```python
from build123d import *

# Parameters (mm, degrees)
BOSS_EXTRUDE2_START = 10
SKETCH3_W           = 70
SKETCH3_H           = 5
BOSS_EXTRUDE2_DEPTH = 120
BOSS_EXTRUDE3_START = 18
BOSS_EXTRUDE3_DEPTH = 8
SKETCH4_R           = 2.1
CUT_EXTRUDE1_DEPTH  = 11
FILLET1_R           = 10
SKETCH5_R           = 1.6
CUT_EXTRUDE2_DEPTH  = 11
CUT_EXTRUDE5_REACH  = 139.915
SKETCH7_R           = 1.6
CUT_EXTRUDE6_REACH  = 139.915
SKETCH6_W           = 40
SKETCH6_H           = 4


with BuildPart() as part:
    # Sketch3 → Boss-Extrude2 (new body)
    with BuildSketch(Plane.XY.offset(BOSS_EXTRUDE2_START)):
        with Locations((0, 11)):
            Rectangle(SKETCH3_W, SKETCH3_H)
    extrude(amount=BOSS_EXTRUDE2_DEPTH)

    # Sketch1 → Boss-Extrude3 (add, symmetric)
    with BuildSketch(Plane.XY.offset(BOSS_EXTRUDE3_START)):
        with BuildLine():
            Line((-14.625621312, 8.5), (14.625621312, 8.5))
            add(Edge.make_bspline(
                [(14.625621312, 8.5), (12.253002272, 8.152861079), (11.086674652, 1.382068579), (9.719671925, -2.351165174)],
                knots=[0, 0, 0, 0, 1, 1, 1, 1], degree=3))
            ThreePointArc((9.719671925, -2.351165174), (9.204012528, -3.909751064), (8.440296287, -5.362965465))
            ThreePointArc((8.440296287, -5.362965465), (7.859364307, -6.648156809), (7.660444431, -8.044448198))
            Line((7.660444431, -8.044448198), (7.660444431, -16.427876097))
            Line((7.660444431, -16.427876097), (6.160444431, -16.427876097))
            Line((6.160444431, -16.427876097), (5.160444431, -16.427876097))
            Line((5.160444431, -16.427876097), (5.160444431, -6.557170147))
            ThreePointArc((5.160444431, -6.557170147), (5.34546922, -4.208445066), (5.895979032, -1.917662968))
            ThreePointArc((5.895979032, -1.917662968), (0, 6.2), (-5.895979032, -1.917662968))
            ThreePointArc((-5.895979032, -1.917662968), (-5.34546922, -4.208445066), (-5.160444431, -6.557170147))
            Line((-5.160444431, -6.557170147), (-5.160444431, -16.427876097))
            Line((-5.160444431, -16.427876097), (-6.160444431, -16.427876097))
            Line((-6.160444431, -16.427876097), (-7.660444431, -16.427876097))
            Line((-7.660444431, -16.427876097), (-7.660444431, -8.044448198))
            ThreePointArc((-7.660444431, -8.044448198), (-7.859364307, -6.648156809), (-8.440296287, -5.362965465))
            ThreePointArc((-8.440296287, -5.362965465), (-9.204012528, -3.909751064), (-9.719671925, -2.351165174))
            add(Edge.make_bspline(
                [(-14.625621312, 8.5), (-12.253002272, 8.152861079), (-11.086674652, 1.382068579), (-9.719671925, -2.351165174)],
                knots=[0, 0, 0, 0, 1, 1, 1, 1], degree=3))
        make_face()
    boss_extrude3 = extrude(amount=BOSS_EXTRUDE3_DEPTH, both=True)

    # Sketch4 → Cut-Extrude1 (cut)
    with BuildSketch(Plane.ZY.offset(7.660444431)):
        with Locations(Location((18, -12.521824291, 0), (0, 0, 270))):
            Circle(SKETCH4_R)
    cut_extrude1 = extrude(amount=-CUT_EXTRUDE1_DEPTH, mode=Mode.SUBTRACT)

    # Mirror2: Boss-Extrude3, Cut-Extrude1 across plane
    add(boss_extrude3.mirror(Plane.XY.offset(70)))
    add(cut_extrude1.mirror(Plane.XY.offset(70)), mode=Mode.SUBTRACT)

    # Fillet1
    fillet1_edges = [part.edges().sort_by_distance(p)[0] for p in [
        (-35, 11, 130),
        (35, 11, 130),
        (-35, 11, 10),
        (35, 11, 10),
    ]]
    fillet(fillet1_edges, radius=FILLET1_R)

    # Sketch5 → Cut-Extrude2 (cut)
    with BuildSketch(Plane(origin=(0, 13.5, 0), x_dir=(1, 0, 0), z_dir=(0, 1, 0))):
        with Locations(Location((29, -25, 0), (0, 0, 270))):
            Circle(SKETCH5_R)
        with Locations(Location((29, -74, 0), (0, 0, 270))):
            Circle(SKETCH5_R)
        with Locations(Location((-29, -74, 0), (0, 0, 270))):
            Circle(SKETCH5_R)
        with Locations(Location((-29, -25, 0), (0, 0, 270))):
            Circle(SKETCH5_R)
    extrude(amount=-CUT_EXTRUDE2_DEPTH, mode=Mode.SUBTRACT)

    # Sketch7 → Cut-Extrude5 (cut, up to next)
    with BuildSketch(Plane(origin=(0, 13.5, 0), x_dir=(1, 0, 0), z_dir=(0, 1, 0)), mode=Mode.PRIVATE) as cut_extrude5_sk1:
        with Locations(Location((12.5, -37, 0), (0, 0, 270))):
            Circle(SKETCH7_R)
    cut_extrude5_tool1 = extrude(cut_extrude5_sk1.sketch, amount=-CUT_EXTRUDE5_REACH, mode=Mode.PRIVATE) & part.part
    # Sketch7 → Cut-Extrude5 (cut, up to next)
    with BuildSketch(Plane(origin=(0, 13.5, 0), x_dir=(1, 0, 0), z_dir=(0, 1, 0)), mode=Mode.PRIVATE) as cut_extrude5_sk2:
        with Locations(Location((12.5, -62, 0), (0, 0, 270))):
            Circle(SKETCH7_R)
    cut_extrude5_tool2 = extrude(cut_extrude5_sk2.sketch, amount=-CUT_EXTRUDE5_REACH, mode=Mode.PRIVATE) & part.part
    # Sketch7 → Cut-Extrude5 (cut, up to next)
    with BuildSketch(Plane(origin=(0, 13.5, 0), x_dir=(1, 0, 0), z_dir=(0, 1, 0)), mode=Mode.PRIVATE) as cut_extrude5_sk3:
        with Locations(Location((-12.5, -62, 0), (0, 0, 270))):
            Circle(SKETCH7_R)
    cut_extrude5_tool3 = extrude(cut_extrude5_sk3.sketch, amount=-CUT_EXTRUDE5_REACH, mode=Mode.PRIVATE) & part.part
    # Sketch7 → Cut-Extrude5 (cut, up to next)
    with BuildSketch(Plane(origin=(0, 13.5, 0), x_dir=(1, 0, 0), z_dir=(0, 1, 0)), mode=Mode.PRIVATE) as cut_extrude5_sk4:
        with Locations(Location((-12.5, -37, 0), (0, 0, 270))):
            Circle(SKETCH7_R)
    cut_extrude5_tool4 = extrude(cut_extrude5_sk4.sketch, amount=-CUT_EXTRUDE5_REACH, mode=Mode.PRIVATE) & part.part
    add(cut_extrude5_tool1.solids().sort_by_distance((12.5, 13.5, 37))[0], mode=Mode.SUBTRACT)
    add(cut_extrude5_tool2.solids().sort_by_distance((12.5, 13.5, 62))[0], mode=Mode.SUBTRACT)
    add(cut_extrude5_tool3.solids().sort_by_distance((-12.5, 13.5, 62))[0], mode=Mode.SUBTRACT)
    add(cut_extrude5_tool4.solids().sort_by_distance((-12.5, 13.5, 37))[0], mode=Mode.SUBTRACT)

    # Sketch6 → Cut-Extrude6 (cut, up to next)
    with BuildSketch(Plane(origin=(0, 13.5, 0), x_dir=(1, 0, 0), z_dir=(0, 1, 0)), mode=Mode.PRIVATE) as cut_extrude6_sk1:
        with Locations((0, -80.5)):
            Rectangle(SKETCH6_W, SKETCH6_H)
    cut_extrude6_tool1 = extrude(cut_extrude6_sk1.sketch, amount=-CUT_EXTRUDE6_REACH, mode=Mode.PRIVATE) & part.part
    # Sketch6 → Cut-Extrude6 (cut, up to next)
    with BuildSketch(Plane(origin=(0, 13.5, 0), x_dir=(1, 0, 0), z_dir=(0, 1, 0)), mode=Mode.PRIVATE) as cut_extrude6_sk2:
        with Locations((0, -109.5)):
            Rectangle(SKETCH6_W, SKETCH6_H)
    cut_extrude6_tool2 = extrude(cut_extrude6_sk2.sketch, amount=-CUT_EXTRUDE6_REACH, mode=Mode.PRIVATE) & part.part
    add(cut_extrude6_tool1.solids().sort_by_distance((0, 13.5, 80.5))[0], mode=Mode.SUBTRACT)
    add(cut_extrude6_tool2.solids().sort_by_distance((0, 13.5, 109.5))[0], mode=Mode.SUBTRACT)


solid = part.part
```
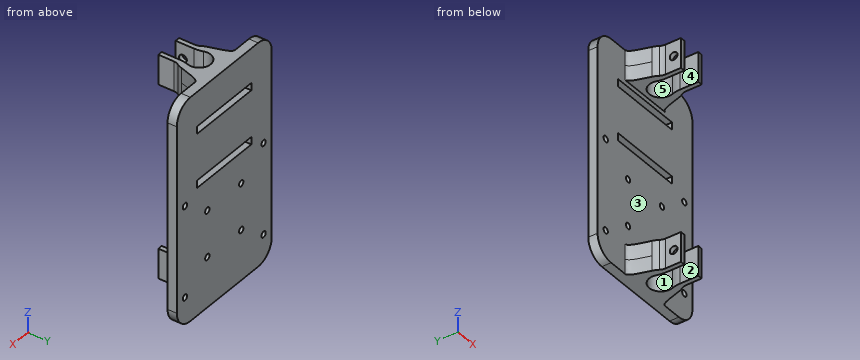
Verification items for the finished model (mm, model axes). Face numbers are marked on the shaded views. A direction names the side the tool comes from. Coordinates: 2 decimals unless noted, no trailing zeros. Order: outer loops, then holes, each group sorted by start corner. A loop starts at its lowest first (then second) coordinate and runs counter-clockwise, first axis right, second up. Notation, with made-up numbers: (-31.5, 4) - (9.5, 4) arc R22 ccw to (9.5, 35) - close; hole circle Ø6 at (-31.75, 82). An arc over 180 degrees is marked (long way). Return JSON: item names as keys, results as strings.
(1) Section check B-B, the plane y = -9.25. Record the cut outline in (x, z).
Filled sheet:
{"outline": "(-7.66, 10) - (-5.16, 10) - (-5.16, 26) - (-7.66, 26) - close; (-7.66, 114) - (-5.16, 114) - (-5.16, 130) - (-7.66, 130) - close; (5.16, 10) - (7.66, 10) - (7.66, 26) - (5.16, 26) - close; (5.16, 114) - (7.66, 114) - (7.66, 130) - (5.16, 130) - close"}
(2) Thickness scan on line 1 along Z through (x, y) = (-0.5, 10); line 2 along X through (y, z) = (9.5, 74); line 3 along X through (y, z) = (10.3, 37). Record the ranges inside material, lowest first.
Filled sheet:
{"line 1": "z = 10 to 78.5, 82.5 to 107.5, 111.5 to 130", "line 2": "x = -35 to -30.6, -27.4 to 27.4, 30.6 to 35", "line 3": "x = -35 to -14.1, -10.9 to 10.9, 14.1 to 35"}
(3) Section check A-A, the plane z = 74. Record the cut outline in (x, y).
Filled sheet:
{"outline": "(-35, 8.5) - (-30.6, 8.5) - (-30.6, 13.5) - (-35, 13.5) - close; (-27.4, 8.5) - (27.4, 8.5) - (27.4, 13.5) - (-27.4, 13.5) - close; (30.6, 8.5) - (35, 8.5) - (35, 13.5) - (30.6, 13.5) - close"}
(4) Section check C-C, the plane x = 29. Record the cut outline in (y, z), and give its area (3 significant figures).
Filled sheet:
{"outline": "(8.5, 10.83) - (13.5, 10.83) - (13.5, 23.4) - (8.5, 23.4) - close; (8.5, 26.6) - (13.5, 26.6) - (13.5, 72.4) - (8.5, 72.4) - close; (8.5, 75.6) - (13.5, 75.6) - (13.5, 129.17) - (8.5, 129.17) - close", "area": "560 mm^2"}
(5) Section check D-D, the plane z = 57. Record the cut outline in (x, y), and give its area (3 significant figures).
Filled sheet:
{"outline": "(-35, 8.5) - (35, 8.5) - (35, 13.5) - (-35, 13.5) - close", "area": "350 mm^2"}
(6) Mould release check, pull along X, two halves, no side actions. Record for the marked faces 1, 2 and 3: pulls with the +X half, pulls with the -X half, needs draft (parallel to the pull), parting line crosses it, or undercut.
Filled sheet:
{"face 1": "undercut", "face 2": "undercut", "face 3": "needs draft"}
(7) Go/stop test with flat-tipped pins: pin 1 (2.5 mm diameter, centred on x = -29, z = 74, fed in from +Y); pin 2 (5.5 mm diameter, centred on y = -12.52, z = 122, fed in from -X); pin 3 (1.5 mm diameter, centred on x = -21, z = 26.5, fed in from -Y); pin 4 (6.5 mm diameter, centred on y = -13.5, z = 21.5, fed in from +X). Record where each tip stops, or that it passes through.
Filled sheet:
{"pin 1": "passes through", "pin 2": "stops at x = -7.66", "pin 3": "stops at y = 8.5", "pin 4": "stops at x = 7.66"}
(8) Access from +Z, -Z, +X, -X, +Y, -Y to the whole of each face (thin tool, end or side, straight path). Record for the marked faces 4 and 5.
Filled sheet:
{"face 4": "+Z, -Z, -Y", "face 5": "+Z, -Z"}
